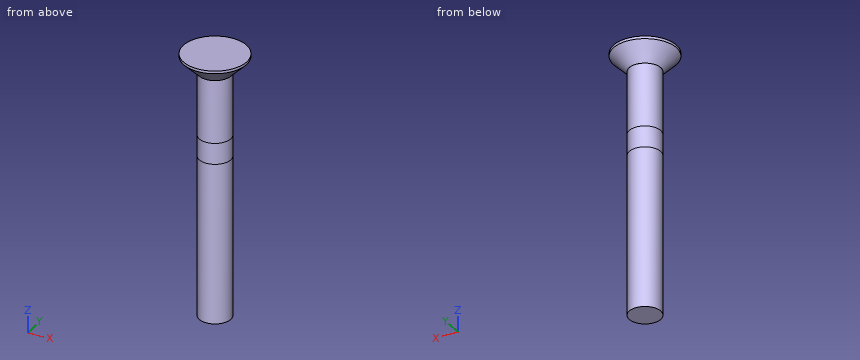
Autodesk Inventor part; units mm, degrees
ref_plane "YZ Plane" through (0, 0, 0) normal (1, 0, 0) x (0, 1, 0)
ref_plane "XZ Plane" through (0, 0, 0) normal (0, 1, 0) x (-1, 0, 0)
ref_plane "XY Plane" through (0, 0, 0) normal (0, 0, 1) x (1, 0, 0)
sketch "スケッチ1" plane through (0, 0, 0) normal (0, 0, 1) x (1, 0, 0)
  circle A0 centre (0, 0) radius 1.5
  dimension "d0" = 3
extrude "押し出し1" add sketch "スケッチ1" along normal blind 6
sketch "スケッチ2" plane through (0, 0, 6) normal (0, 0, 1) x (1, 0, 0)
  circle A0 centre (0, 0) radius 1.5
  circle A1 centre (0, 0) radius 3
  dimension "d3" = 6
extrude "押し出し2" add sketch "スケッチ2" along normal blind 1.75 contours A0 | A1
thread "ねじ1"
chamfer "面取り1" distance 1.5 angle 45 1 edges at (-3, 0, 6)
sketch "スケッチ4" plane through (0, 0, 0) normal (0, 0, -1) x (-1, 0, 0)
  circle A0 centre (0, 0) radius 1.5
extrude "押し出し4" add sketch "スケッチ4" along normal blind 4
sketch "スケッチ5" plane through (0, 0, -4) normal (0, 0, -1) x (-1, 0, 0)
  circle A0 centre (0, 0) radius 1.5
extrude "押し出し5" cut sketch "スケッチ5" against normal blind 2
sketch "スケッチ6" plane through (0, 0, -2) normal (0, 0, -1) x (-1, 0, 0)
  circle A0 centre (0, 0) radius 1.5
extrude "押し出し6" add sketch "スケッチ6" along normal blind 15.25
properties part number "SB　25mm皿ネジ" material "Steel, Mild"
Model file for the job. Use its own axes, mm. Coordinates: 2 decimals unless noted, no trailing zeros. Write each loop counter-clockwise with the first axis right and the second up, starting at its lowest first coordinate (ties: lowest second). Pieces come first, ordered by that corner, then holes. Notation, with made-up numbers: (-37.75, 14.5) - (9.25, 14.5) arc R21 ccw to (9.25, 39.5) - close; hole circle Ø1 at (-5.75, -6.5). An arc over 180 degrees is marked (long way). Use a Markdown table: item, result. Add a question column.
Item 1: Drop a flat-ended pin along its axis: pin 1 (2 mm diameter, centred on x = -2, y = 2, fed in from -Z). Give the stop position or say it passes through.
Item 2: Drill centre lines: line 1 along Y through (x, z) = (-0.1, 0.5); line 2 along X through (y, z) = (1.25, -5.25); line 3 along Y through (x, z) = (-0.85, -14.25). Where is each one in solid material? Low to high.
Item 3: Band-saw the part on C-C, the plane z = -12. Write the cut outline in (x, y).
A:
| question | item | result |
|---|---|---|
| 1 | pin 1 | stops at z = 6.33 |
| 2 | line 1 | y = -1.5 to 1.5 |
| 2 | line 2 | x = -0.83 to 0.83 |
| 2 | line 3 | y = -1.24 to 1.24 |
| 3 | outline | circle Ø3 at (0, 0) |
